Can you work these out from the model? Positions are in its coordinate system, mm. A direction names the side the tool comes from. Round coordinates to 2 decimals unless told otherwise and drop trailing zeros. Loops run counter-clockwise (first coordinate to the right, second up) from the corner with the lowest first, then second, coordinate; pieces in that order, holes last. Notation, with made-up numbers: M -14,45 L 19,45 A15 cw 19,60 Z; hole C 54,-28 d2. An arc over 180 degrees is marked long. Return JSON: item names as keys, results as strings.
```python
from build123d import *

# Parameters (mm, degrees)
SKETCH_1_W          = 25
SKETCH_1_H          = 55
SKETCH_1_W_2        = 90
SKETCH_1_H_2        = 10
EXTRUDE_1_DEPTH     = 15
SKETCH_2_W          = 90
SKETCH_2_H          = 10
EXTRUDE_2_DEPTH     = 20
CHAMFER_4_SIZE      = 10
SKETCH_4_R          = 2
CUT_EXTRUDE_1_DEPTH = 11
SKETCH_5_R          = 3.5
CUT_EXTRUDE_2_DEPTH = 7


with BuildPart() as part:
    # 草圖1 → 填料-伸長1 (new body)
    with BuildSketch(Plane.XY):
        with BuildLine():
            Line((-62.370495495, 24.5), (-30.870495495, 24.5))
            Line((-30.870495495, 24.5), (-5.870495495, 24.5))
            Line((-5.870495495, 24.5), (25.629504505, 24.5))
            Line((25.629504505, 24.5), (25.629504505, 74.5))
            Line((25.629504505, 74.5), (19.129504505, 74.5))
            ThreePointArc((19.129504505, 74.5), (-18.370495495, 37), (-55.870495495, 74.5))
            Line((-55.870495495, 74.5), (-62.370495495, 74.5))
            Line((-62.370495495, 74.5), (-62.370495495, 24.5))
        make_face()
        with Locations((-18.370495495, -3)):
            Rectangle(SKETCH_1_W, SKETCH_1_H)
        with Locations((-18.370495495, -35.5)):
            Rectangle(SKETCH_1_W_2, SKETCH_1_H_2)
    extrude(amount=EXTRUDE_1_DEPTH)

    # 草圖2 → 填料-伸長2 (add)
    with BuildSketch(Plane.XY.offset(15)):
        with Locations((-18.370495495, -35.5)):
            Rectangle(SKETCH_2_W, SKETCH_2_H)
    extrude(amount=EXTRUDE_2_DEPTH)

    # 導角4
    chamfer_4_edges = [part.edges().sort_by_distance(p)[0] for p in [
        (-5.870495495, -30.5, 7.5),
        (-30.870495495, -30.5, 7.5),
        (-18.370495495, -30.5, 15),
    ]]
    chamfer(chamfer_4_edges, length=CHAMFER_4_SIZE)

    # 草圖4 → 除料-伸長1 (cut, through all)
    with BuildSketch(Plane(origin=(0, -30.5, 0), x_dir=(1, 0, 0), z_dir=(0, 1, 0))):
        with Locations((-53.370495495, -20)):
            Circle(SKETCH_4_R)
        with Locations((16.629504505, -20)):
            Circle(SKETCH_4_R)
    extrude(amount=-CUT_EXTRUDE_1_DEPTH, mode=Mode.SUBTRACT)

    # 草圖5 → 除料-伸長2 (cut)
    with BuildSketch(Plane(origin=(0, -30.5, 0), x_dir=(1, 0, 0), z_dir=(0, 1, 0))):
        with Locations((-53.370495495, -20)):
            Circle(SKETCH_5_R)
        with Locations((16.629504505, -20)):
            Circle(SKETCH_5_R)
    extrude(amount=-CUT_EXTRUDE_2_DEPTH, mode=Mode.SUBTRACT)


solid = part.part
```
Q1. Suppose I cut it at C-C, the plane x = -54. Please give me the cut outline in (y, z), plus the area to 3 significant figures.
Results:
{"outline": "M -40.5,0 L -30.5,0 L -30.5,16.56 L -37.5,16.56 L -37.5,18.1 L -40.5,18.1 Z; M -40.5,21.9 L -37.5,21.9 L -37.5,23.44 L -30.5,23.44 L -30.5,35 L -40.5,35 Z; M 24.5,0 L 62.8,0 L 62.8,15 L 24.5,15 Z", "area": "865 mm2"}
Q2. If I drill on line 1 along X through (y, z) = (-35, 20); line 2 along X through (y, z) = (-39.8, 20); line 3 along Z through (x, y) = (22, 39.5), over which ranges is the centre line in solid material (lowest first)?
Results:
{"line 1": "x = -63.37 to -56.87, -49.87 to 13.13, 20.13 to 26.63", "line 2": "x = -63.37 to -55.37, -51.37 to 14.63, 18.63 to 26.63", "line 3": "z = 0 to 15"}
Q3. Suppose I cut it at D-D, the plane x = -36. Please give me the cut outline in (y, z), plus the area to 3 significant figures.
Results:
{"outline": "M -40.5,0 L -25.63,0 L -25.63,20.13 L -30.5,25 L -30.5,35 L -40.5,35 Z; M 24.5,0 L 41.4,0 L 41.4,15 L 24.5,15 Z", "area": "713 mm2"}
Q4. On a 3-axis mill with a long thin cutter (end or side, diameter ignored), from which of +Z, -Z, +X, -X, +Y, -Y can I reach the whole of each face in a straight line? I mean faces 4 (the flat face through (-47, 24.5, 7)), 5 (the cylindrical face through (18.51, -33.95, 17.05)), 6 (the flat face through (-5.87, 2, 7)), 7 (the flat face through (-62.37, 50, 7)), 8 (the flat face through (-19, 28, 15)). Say none if no direction works.
Results:
{"face 4": "+Z, -Z, -X", "face 5": "+Y", "face 6": "+Z, -Z, +X", "face 7": "+Z, -Z, -X, +Y", "face 8": "+Z, +X, -X, +Y"}
Q5. I'm going to push flat-ended pins straight in: pin 1 Ø8 at (x, z) = (-53.37, 20) entering from +Y; pin 2 Ø10 at (x, z) = (-24, 5.5) entering from +Y; pin 3 Ø6 at (x, y) = (-3.5, 37) entering from -Z; pin 4 Ø8 at (x, z) = (5, 16.5) entering from +Y. Where does each tip first touch, or does it pass through?
Results:
{"pin 1": "stops at y = -30.5", "pin 2": "stops at y = 38.54", "pin 3": "stops at z = 0", "pin 4": "stops at y = 48.56"}
Q6. Suppose I cut it at A-A, the plane y = 65.5. Please give me the cut outline in (x, z), plus the area to 3 significant figures.
Results:
{"outline": "M -62.37,0 L -54.77,0 L -54.77,15 L -62.37,15 Z; M 18.03,0 L 25.63,0 L 25.63,15 L 18.03,15 Z", "area": "228 mm2"}
Q7. Suppose I cut it at B-B, the plane z = 2.5. Please give me the cut outline in (x, y).
Results:
{"outline": "M -63.37,-40.5 L 26.63,-40.5 L 26.63,-30.5 L 4.13,-30.5 L -5.87,-20.5 L -5.87,24.5 L 25.63,24.5 L 25.63,74.5 L 19.13,74.5 A37.5 cw -55.87,74.5 L -62.37,74.5 L -62.37,24.5 L -30.87,24.5 L -30.87,-20.5 L -40.87,-30.5 L -63.37,-30.5 Z"}
Q8. Thinking about a two-plate mould opening in Y: for faces 1 (the flat face through (10, 24.5, 7)), 2 (the flat face through (-18.7, -25.6, 20.1)), 3 (the cylindrical face through (17.7, -38.98, 18.31)), which applies, pulls with the +Y half, pulls with the -Y half, needs draft (parallel to the pull), parting line crosses it, or undercut?
Results:
{"face 1": "undercut", "face 2": "pulls with the +Y half", "face 3": "needs draft"}
